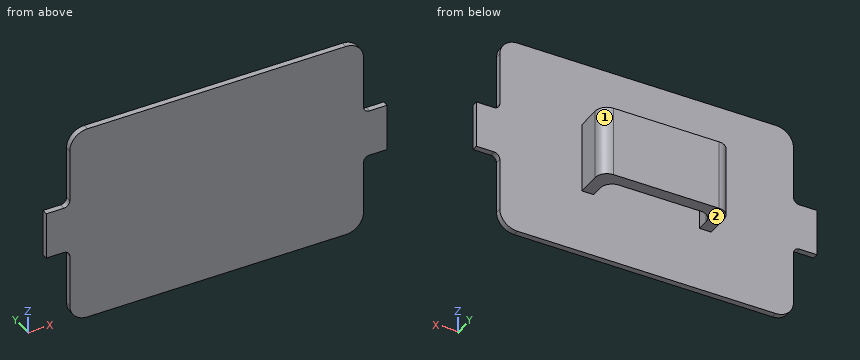
```python
from build123d import *

# Parameters (mm, degrees)
SKETCH1_W           = 125
SKETCH1_H           = 85
BOSS_EXTRUDE1_DEPTH = 2.5
SKETCH2_W           = 10
SKETCH2_H           = 20
SKETCH2_H_2         = 10
BOSS_EXTRUDE2_DEPTH = 2.5
FILLET1_R           = 2.5
FILLET2_R           = 7.5
SKETCH3_W           = 5
SKETCH3_H           = 15
BOSS_EXTRUDE3_DEPTH = 15
BOSS_EXTRUDE4_REACH = 130.671
SKETCH4_W           = 30
SKETCH4_H           = 5
FILLET3_R           = 5


with BuildPart() as part:
    # Sketch1 → Boss-Extrude1 (new body)
    with BuildSketch(Plane(origin=(0, 0, 0), x_dir=(1, 0, 0), z_dir=(0, 1, 0))):
        with Locations((62.5, 42.5)):
            Rectangle(SKETCH1_W, SKETCH1_H)
    extrude(amount=BOSS_EXTRUDE1_DEPTH)

    # Sketch2 → Boss-Extrude2 (add)
    with BuildSketch(Plane(origin=(0, 2.5, 0), x_dir=(1, 0, 0), z_dir=(0, 1, 0))):
        with Locations((130, 42.5)):
            Rectangle(SKETCH2_W, SKETCH2_H)
        with Locations((-5, 37.5)):
            Rectangle(SKETCH2_W, SKETCH2_H_2)
        with Locations((-5, 47.5)):
            Rectangle(SKETCH2_W, SKETCH2_H_2)
    extrude(amount=-BOSS_EXTRUDE2_DEPTH)

    # Fillet1
    fillet1_edges = [part.edges().sort_by_distance(p)[0] for p in [
        (125, 1.25, -32.5),
        (125, 1.25, -52.5),
        (0, 1.25, -32.5),
        (0, 1.25, -52.5),
    ]]
    fillet(fillet1_edges, radius=FILLET1_R)

    # Fillet2
    fillet2_edges = [part.edges().sort_by_distance(p)[0] for p in [
        (0, 1.25, -85),
        (125, 1.25, -85),
        (125, 1.25, 0),
        (0, 1.25, 0),
    ]]
    fillet(fillet2_edges, radius=FILLET2_R)

    # Sketch3 → Boss-Extrude3 (add)
    with BuildSketch(Plane(origin=(0, 2.5, 0), x_dir=(1, 0, 0), z_dir=(0, 1, 0))):
        with Locations((37.5, 50)):
            Rectangle(SKETCH3_W, SKETCH3_H)
        with Locations((37.5, 35)):
            Rectangle(SKETCH3_W, SKETCH3_H)
        with Locations((87.5, 50)):
            Rectangle(SKETCH3_W, SKETCH3_H)
        with Locations((87.5, 35)):
            Rectangle(SKETCH3_W, SKETCH3_H)
    extrude(amount=BOSS_EXTRUDE3_DEPTH)

    # Sketch4 → Boss-Extrude4 (add, up to next)
    with BuildSketch(Plane(origin=(40, 0, 0), x_dir=(0, 0, -1), z_dir=(1, 0, 0)), mode=Mode.PRIVATE) as boss_extrude4_sk1:
        with Locations((42.5, 15)):
            Rectangle(SKETCH4_W, SKETCH4_H)
    boss_extrude4_tool1 = extrude(boss_extrude4_sk1.sketch, amount=BOSS_EXTRUDE4_REACH, mode=Mode.PRIVATE) - part.part
    add(boss_extrude4_tool1.solids().sort_by_distance((40, 15, -42.5))[0])

    # Fillet3
    fillet3_edges = [part.edges().sort_by_distance(p)[0] for p in [
        (35, 17.5, -42.5),
        (90, 17.5, -42.5),
        (85, 12.5, -42.5),
        (40, 12.5, -42.5),
    ]]
    fillet(fillet3_edges, radius=FILLET3_R)


solid = part.part
```
Input: part model. Units: mm. Frame: model coordinates. Face numbers are marked on the shaded views. Coordinates: 2 decimals unless noted, no trailing zeros. Write each loop counter-clockwise with the first axis right and the second up, starting at its lowest first coordinate (ties: lowest second). Pieces come first, ordered by that corner, then holes. Notation, with made-up numbers: (26.5, 26.5) -> (82.5, 26.5) arc R29 cw to (82.5, 56.5) -> close; hole circle Ø2 at (35.5, 12). An arc over 180 degrees is marked (long way). Write each question's results on one line, items separated by ' | '.
Item 1: Mould query, pull axis X, two halves, no side actions, for the marked faces 1 and 2. Classes: +X half, -X half, draft (parallel to the pull), parting line (faces both ways), or undercut.
Conclusion:
face 1: +X half | face 2: draft
Item 2: Section query B-B on y = 5. Return loops of the section in (x, z).
Conclusion:
outline: (35, -57.5) -> (40, -57.5) -> (40, -27.5) -> (35, -27.5) -> close; (85, -57.5) -> (90, -57.5) -> (90, -27.5) -> (85, -27.5) -> close
Item 3: Section query C-C on z = -39. Return loops of the section in (x, y).
Conclusion:
outline: (-10, 0) -> (135, 0) -> (135, 2.5) -> (90, 2.5) -> (90, 12.5) arc R5 ccw to (85, 17.5) -> (40, 17.5) arc R5 ccw to (35, 12.5) -> (35, 2.5) -> (-10, 2.5) -> close; hole (40, 2.5) -> (85, 2.5) -> (85, 7.5) arc R5 ccw to (80, 12.5) -> (45, 12.5) arc R5 ccw to (40, 7.5) -> close
Item 4: Section query A-A on x = 71. Return loops of the section in (y, z), plus the area to 4 significant figures.
Conclusion:
outline: (0, -85) -> (2.5, -85) -> (2.5, 0) -> (0, 0) -> close; (12.5, -57.5) -> (17.5, -57.5) -> (17.5, -27.5) -> (12.5, -27.5) -> close | area: 362.5 mm^2
Item 5: Section query D-D on z = -13. Return loops of the section in (x, y).
Conclusion:
outline: (0, 0) -> (125, 0) -> (125, 2.5) -> (0, 2.5) -> close
Item 6: Material intervals for probe 1 along X at (y, z) = (5.5, -35); probe 2 along Y at (x, z) = (8.5, -77.5); probe 3 along Z at (x, y) = (66, 15.5), sorted ascending.
Conclusion:
probe 1: x = 35 to 40, 85 to 90 | probe 2: y = 0 to 2.5 | probe 3: z = -57.5 to -27.5
Item 7: Pin query (flat end, axial travel): pin 1 Ø1.2 at (y, z) = (1, -61) entering from -X; pin 2 Ø3 at (y, z) = (1.5, -65.5) entering from +X; pin 3 Ø1.2 at (x, y) = (-8, 1) entering from +Z; pin 4 Ø3 at (x, y) = (73.5, 4.5) entering from +Z. Return the tip coordinate at first contact, or that it passes through.
Conclusion:
pin 1: stops at x = 0 | pin 2: stops at x = 125 | pin 3: stops at z = -32.5 | pin 4: passes through
